Here's the drawing with two shaded views (mm, measured from the low corner). I have some questions. A direction names the side the tool comes from. Coordinates: 2 decimals unless noted, no trailing zeros. Write each loop counter-clockwise with the first axis right and the second up, starting at its lowest first coordinate (ties: lowest second). Pieces come first, ordered by that corner, then holes.
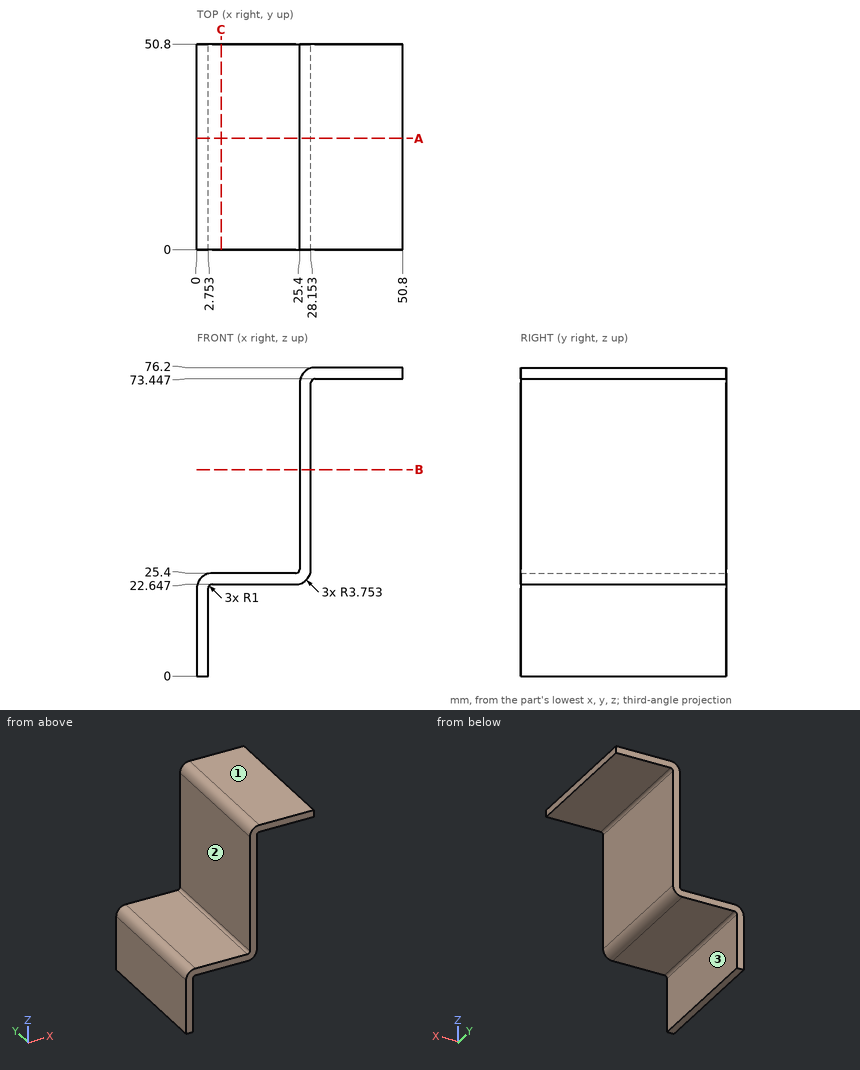
1. For pin 1 (4 mm diameter, centred on y = 18.5, z = 28.5, fed in from -X); pin 2 (1 mm diameter, centred on y = 28.5, z = 15, fed in from +X); pin 3 (10.5 mm diameter, centred on x = 13, y = 21, fed in from +Z); pin 4 (5 mm diameter, centred on x = 9, z = 25, fed in from -Y), each with a flat end and sliding along its axis, tell me the tip position at first contact or that it passes through.
Verdict:
pin 1: stops at x = 25.4
pin 2: stops at x = 2.75
pin 3: stops at z = 25.4
pin 4: stops at y = 0
2. Please list where these lines run through material, in increasing order: line 1 along Z through (x, y) = (16, 9.5); line 2 along X through (y, z) = (16, 55); line 3 along X through (y, z) = (4, 15.5).
Verdict:
line 1: z = 22.65 to 25.4
line 2: x = 25.4 to 28.15
line 3: x = 0 to 2.75
3. I want a section at C-C on x = 6. Please give me the cut outline in (y, z), plus the area to 3 significant figures.
Verdict:
outline: (0, 22.65) - (50.8, 22.65) - (50.8, 25.4) - (0, 25.4) - close
area: 140 mm2
4. I want a section at A-A on y = 27.5. Please give me the cut outline in (x, z).
Verdict:
outline: (0, 0) - (2.75, 0) - (2.75, 21.65) arc R1 cw to (3.75, 22.65) - (24.4, 22.65) arc R3.75 ccw to (28.15, 26.4) - (28.15, 72.45) arc R1 cw to (29.15, 73.45) - (50.8, 73.45) - (50.8, 76.2) - (29.15, 76.2) arc R3.75 ccw to (25.4, 72.45) - (25.4, 26.4) arc R1 cw to (24.4, 25.4) - (3.75, 25.4) arc R3.75 ccw to (0, 21.65) - close
5. On a 3-axis mill with a long thin cutter (end or side, diameter ignored), from which of +Z, -Z, +X, -X, +Y, -Y can I reach the whole of each face in a straight line? I mean the marked faces 1, 2 and 3. Say none if no direction works.
Verdict:
face 1: +Z, +X, -X, +Y, -Y
face 2: +Z, -X, +Y, -Y
face 3: -Z, +X, +Y, -Y
6. I want a section at B-B on z = 51. Please give me the cut outline in (x, y), plus the area to 3 significant figures.
Verdict:
outline: (25.4, 0) - (28.15, 0) - (28.15, 50.8) - (25.4, 50.8) - close
area: 140 mm2
